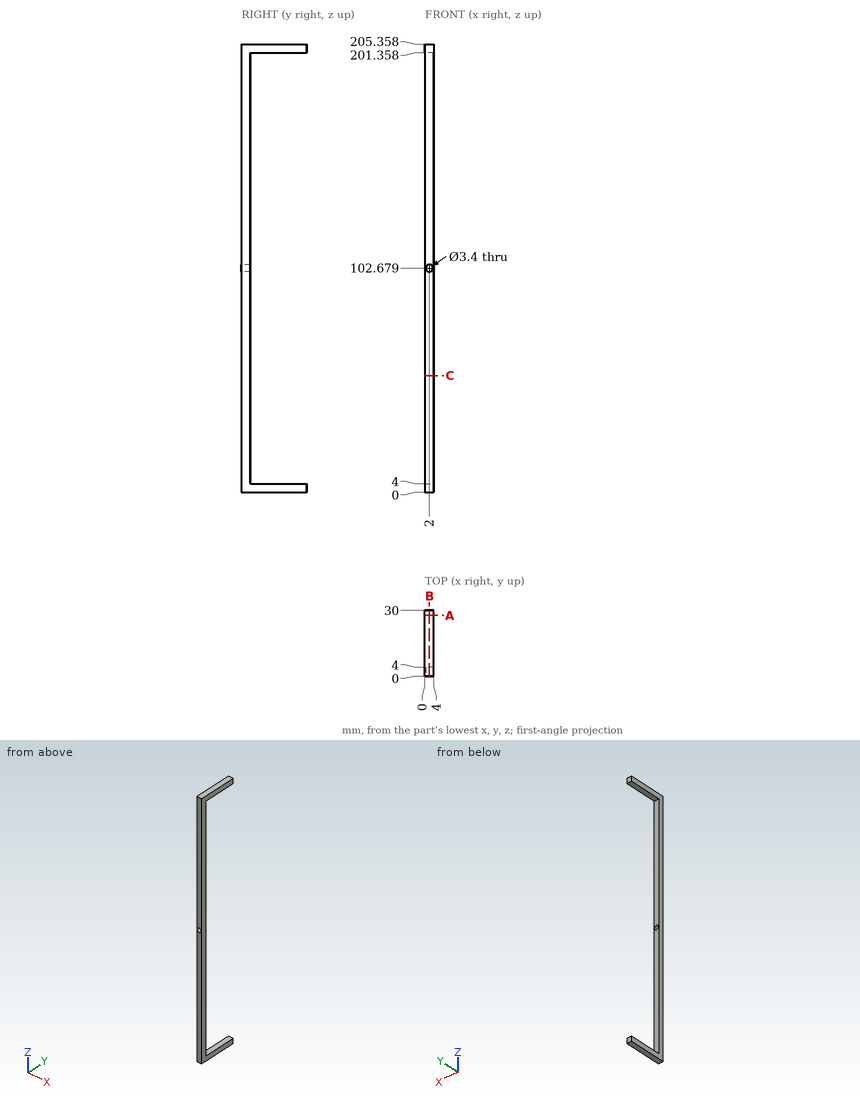
Design review of the part shown in the three views and the two pictorial views. Dimensions are in mm from the part's minimum x, y and z. Round coordinates to 2 decimals unless told otherwise and drop trailing zeros. Order: outer loops, then holes, each group sorted by start corner. A loop starts at its lowest first (then second) coordinate and runs counter-clockwise, first axis right, second up. Notation, with made-up numbers: (11, 31.5) -> (35, 31.5) arc R11 cw to (35, 50.5) -> close; hole circle Ø5 at (-12, 21). An arc over 180 degrees is marked (long way). Write item = value, one per line. Start each with the question number.
1) To check wall thickness, follow line 1 (Z direction, x = 2, y = 1.6); line 2 (Z direction, x = 3.5, y = 17.25); line 3 (Y direction, x = 3.3, z = 140). State the ranges of each line that lie inside material, in increasing order. Write a range as from..to.
2) Take a section at C-C on z = 53.5. State the section outline as (x, y) points, plus the area to 3 significant figures.
3) Insertion check: pin 1 (2 mm diameter, centred on x = 3.5, z = 115, fed in from +Y); pin 2 (2 mm diameter, centred on y = 3.5, z = 143, fed in from -X). Each pin has a flat end and moves straight along its axis. Give the tip position at first contact, or say it passes through.
4) Take a section at A-A on y = 27.75. State the section outline as (x, z) points.
5) Take a section at B-B on x = 2. State the section outline as (y, z) points.
Verdict:
q1.line_1 = 0..100.98, 104.38..205.36
q1.line_2 = 0..4, 201.36..205.36
q1.line_3 = 0..4
q2.outline = (0, 0) -> (4, 0) -> (4, 4) -> (0, 4) -> close
q2.area = 16.0 mm2
q3.pin_1 = 4
q3.pin_2 = 0
q4.outline = (0, 0) -> (4, 0) -> (4, 4) -> (0, 4) -> close; (0, 201.36) -> (4, 201.36) -> (4, 205.36) -> (0, 205.36) -> close
q5.outline = (0, 0) -> (30, 0) -> (30, 4) -> (4, 4) -> (4, 100.98) -> (0, 100.98) -> close; (0, 104.38) -> (4, 104.38) -> (4, 201.36) -> (30, 201.36) -> (30, 205.36) -> (0, 205.36) -> close
